```python
from build123d import *

# Parameters (mm, degrees)
EXTRUDE2_DEPTH               = 25.4
SKETCH3_W                    = 125
SKETCH3_H                    = 125
EXTRUDE3_DEPTH               = 153.67
SKETCH4_W                    = 100
SKETCH4_H                    = 100
CUT_EXTRUDE1_DEPTH           = 153.67
SKETCH5_W                    = 74.2
SKETCH5_H                    = 76.2
CUT_EXTRUDE2_DEPTH           = 305.913618751
SKETCH6_W                    = 74.2
SKETCH6_H                    = 76.2
CUT_EXTRUDE3_DEPTH           = 305.913618751
HOLE_WIZARD_M6_3_D           = 5
HOLE_WIZARD_M6_3_DEPTH       = 15
HOLE_WIZARD_M6_3_CBORE_D     = 6
HOLE_WIZARD_M6_3_CBORE_DEPTH = 12
HOLE_WIZARD_M6_3_TIP         = 1.502151548
HOLE_WIZARD_1_D              = 6.6
HOLE_WIZARD_1_CBORE_D        = 11
HOLE_WIZARD_1_CBORE_DEPTH    = 6.8
HOLE_WIZARD_M6_2_D           = 6
LPATTERN2_COUNT              = 4
LPATTERN2_PITCH              = 25
LPATTERN2_COUNT_DIR2         = 4
LPATTERN2_PITCH_DIR2         = 25


with BuildPart() as part:
    # Sketch2 → Extrude2 (new body)
    with BuildSketch(Plane(origin=(0, 0, 0), x_dir=(1, 0, 0), z_dir=(0, 1, 0))):
        with BuildLine():
            Line((15, 0), (175, 0))
            ThreePointArc((175, 0), (185.606601718, 4.393398282), (190, 15))
            Line((190, 15), (190, 175))
            ThreePointArc((190, 175), (185.606601718, 185.606601718), (175, 190))
            Line((175, 190), (15, 190))
            ThreePointArc((15, 190), (4.393398282, 185.606601718), (0, 175))
            Line((0, 175), (0, 15))
            ThreePointArc((0, 15), (4.393398282, 4.393398282), (15, 0))
        make_face()
    extrude(amount=EXTRUDE2_DEPTH)

    # Sketch3 → Extrude3 (add)
    with BuildSketch(Plane(origin=(0, 25.4, 0), x_dir=(-1, 0, 0), z_dir=(0, 1, 0))):
        with Locations((-95, -95)):
            Rectangle(SKETCH3_W, SKETCH3_H)
    extrude(amount=EXTRUDE3_DEPTH)

    # Sketch4 → Cut-Extrude1 (cut)
    with BuildSketch(Plane(origin=(0, 179.07, 0), x_dir=(-1, 0, 0), z_dir=(0, 1, 0))):
        with Locations((-95, -95)):
            Rectangle(SKETCH4_W, SKETCH4_H)
    extrude(amount=-CUT_EXTRUDE1_DEPTH, mode=Mode.SUBTRACT)

    # Sketch5 → Cut-Extrude2 (cut, through all)
    with BuildSketch(Plane.XY.offset(-32.5)):
        Polygon((45.6085824, 179.07), (144.3914176, 179.07), (95, 129.6785824), align=None)
        with Locations((95, 63.5)):
            Rectangle(SKETCH5_W, SKETCH5_H)
    extrude(amount=-CUT_EXTRUDE2_DEPTH, mode=Mode.SUBTRACT)

    # Sketch6 → Cut-Extrude3 (cut, through all)
    with BuildSketch(Plane(origin=(157.5, 0, 0), x_dir=(0, 0, -1), z_dir=(1, 0, 0))):
        Polygon((45.6085824, 179.07), (144.3914176, 179.07), (95, 129.6785824), align=None)
        with Locations((95, 63.5)):
            Rectangle(SKETCH6_W, SKETCH6_H)
    extrude(amount=-CUT_EXTRUDE3_DEPTH, mode=Mode.SUBTRACT)

    # M6 螺纹孔3
    with Locations(Plane(origin=(0, 179.07, 0), x_dir=(-1, 0, 0), z_dir=(0, 1, 0))):
        with Locations((-151.5, -151.5), (-151.5, -38.5), (-38.5, -38.5), (-38.5, -151.5)):
            CounterBoreHole(HOLE_WIZARD_M6_3_D / 2, HOLE_WIZARD_M6_3_CBORE_D / 2, HOLE_WIZARD_M6_3_CBORE_DEPTH, depth=HOLE_WIZARD_M6_3_DEPTH)
            with Locations((0, 0, -(HOLE_WIZARD_M6_3_DEPTH + HOLE_WIZARD_M6_3_TIP / 2))):  # 118° drill point
                Cone(0, HOLE_WIZARD_M6_3_D / 2, HOLE_WIZARD_M6_3_TIP, mode=Mode.SUBTRACT)

    # 打孔尺寸(%根据)内六角圆柱头螺钉的类型1 (through all)
    with Locations(Plane(origin=(0, 25.4, 0), x_dir=(-1, 0, 0), z_dir=(0, 1, 0))):
        with Locations((-170, -20), (-170, -170), (-20, -170), (-20, -20)):
            CounterBoreHole(HOLE_WIZARD_1_D / 2, HOLE_WIZARD_1_CBORE_D / 2, HOLE_WIZARD_1_CBORE_DEPTH)

    # M6 螺纹孔2 (through all)
    with Locations(Plane(origin=(0, 25.4, 0), x_dir=(-1, 0, 0), z_dir=(0, 1, 0))):
        with Locations((-57.5, -132.5)):
            hole_wizard_m6_2 = Hole(HOLE_WIZARD_M6_2_D / 2)

    # LPattern2: Hole Wizard M6 _2 4 × 4
    with Locations(*[(i * LPATTERN2_PITCH, 0, j * LPATTERN2_PITCH_DIR2) for i in range(LPATTERN2_COUNT) for j in range(LPATTERN2_COUNT_DIR2) if (i, j) != (0, 0)]):
        add(hole_wizard_m6_2, mode=Mode.SUBTRACT)


solid = part.part
```
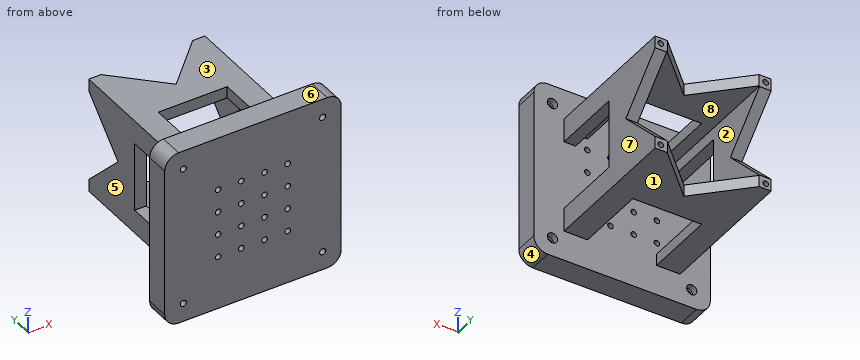
Check sheet for the modelled part. Datum: model origin and axes. Units: mm. Face numbers are marked on the shaded views. A direction names the side the tool comes from. Coordinates: 2 decimals unless noted, no trailing zeros. Loops run counter-clockwise (first coordinate to the right, second up) from the corner with the lowest first, then second, coordinate; pieces in that order, holes last. Notation, with made-up numbers: M 82.5,-37 L 123.5,-37 A24 ccw 123.5,-9 Z; hole C 50.25,-20.5 d6. An arc over 180 degrees is marked long. Answer as a JSON object with one key per item and string values.
1. Sectioned sample at B-B on z = -170. Record the cut outline in (x, y).
Outcome:
{"outline": "M 0,0 L 16.7,0 L 16.7,18.6 L 14.5,18.6 L 14.5,25.4 L 0,25.4 Z; M 23.3,0 L 166.7,0 L 166.7,18.6 L 164.5,18.6 L 164.5,25.4 L 25.5,25.4 L 25.5,18.6 L 23.3,18.6 Z; M 173.3,0 L 190,0 L 190,25.4 L 175.5,25.4 L 175.5,18.6 L 173.3,18.6 Z"}
2. Sectioned sample at C-C on x = 88.5. Record the cut outline in (y, z), and give its area (3 significant figures).
Outcome:
{"outline": "M 0,-190 L 25.4,-190 L 25.4,0 L 0,0 Z; M 101.6,-157.5 L 136.18,-157.5 L 136.18,-145 L 101.6,-145 Z; M 101.6,-45 L 136.18,-45 L 136.18,-32.5 L 101.6,-32.5 Z", "area": "5,690 mm²"}
3. Scan lines: L1, parallel to X at y = 15.25, z = -132.5; L2, parallel to X at y = 5, z = -170; L3, parallel to Z at x = 132.5, y = 18. Record each from-to range of solid material in increasing order. Write a range as from..to.
Outcome:
{"L1": "0..54.5, 60.5..79.5, 85.5..104.5, 110.5..129.5, 135.5..190", "L2": "0..16.7, 23.3..166.7, 173.3..190", "L3": "-190..-135.5, -129.5..-110.5, -104.5..-85.5, -79.5..-60.5, -54.5..0"}
4. Sectioned sample at A-A on y = 38. Record the cut outline in (x, z).
Outcome:
{"outline": "M 32.5,-157.5 L 57.9,-157.5 L 57.9,-145 L 45,-145 L 45,-132.1 L 32.5,-132.1 Z; M 32.5,-57.9 L 45,-57.9 L 45,-45 L 57.9,-45 L 57.9,-32.5 L 32.5,-32.5 Z; M 132.1,-157.5 L 157.5,-157.5 L 157.5,-132.1 L 145,-132.1 L 145,-145 L 132.1,-145 Z; M 132.1,-45 L 145,-45 L 145,-57.9 L 157.5,-57.9 L 157.5,-32.5 L 132.1,-32.5 Z"}
5. Release check for a two-part mould opening along Z. For the marked faces 6, 7 and 8 record: pulls with the +Z half, pulls with the -Z half, needs draft (parallel to the pull), parting line crosses it, or undercut.
Outcome:
{"face 6": "pulls with the +Z half", "face 7": "needs draft", "face 8": "undercut"}
6. Access from +Z, -Z, +X, -X, +Y, -Y to the whole of each face (thin tool, end or side, straight path). Record for the marked faces 1, 2, 3, 4 and 5.
Outcome:
{"face 1": "-Z, +X, -X, +Y", "face 2": "+Y", "face 3": "+Z, +X, -X, +Y", "face 4": "-Z, +X, +Y, -Y", "face 5": "+Z, -Z, -X, +Y"}
7. Depth check by flat-ended pin: P1, Ø2, axis at y = 35.5, z = -149, coming from the +X side; P2, Ø6, axis at y = 70, z = -37.5, coming from the -X side; P3, Ø9.5, axis at x = 107.5, z = -132.5, coming from the +Y side. Enter the tip coordinate at first touch or a pass-through.
Outcome:
{"P1": "x = 157.5", "P2": "x = 32.5", "P3": "y = 25.4"}
8. Sectioned sample at D-D on x = 107.5. Record the cut outline in (y, z).
Outcome:
{"outline": "M 0,-190 L 25.4,-190 L 25.4,-135.5 L 0,-135.5 Z; M 0,-129.5 L 25.4,-129.5 L 25.4,-110.5 L 0,-110.5 Z; M 0,-104.5 L 25.4,-104.5 L 25.4,-85.5 L 0,-85.5 Z; M 0,-79.5 L 25.4,-79.5 L 25.4,-60.5 L 0,-60.5 Z; M 0,-54.5 L 25.4,-54.5 L 25.4,0 L 0,0 Z; M 101.6,-157.5 L 142.18,-157.5 L 142.18,-145 L 101.6,-145 Z; M 101.6,-45 L 142.18,-45 L 142.18,-32.5 L 101.6,-32.5 Z"}
